Input: part model. Units: mm. Frame: model coordinates. A direction names the side the tool comes from. Coordinates: 2 decimals unless noted, no trailing zeros. Write each loop counter-clockwise with the first axis right and the second up, starting at its lowest first coordinate (ties: lowest second). Pieces come first, ordered by that corner, then holes.
from build123d import *

# Parameters (mm, degrees)
SKETCH_1_R          = 30.47
EXTRUDE_1_DEPTH     = 13
SKETCH_2_R          = 33.47
EXTRUDE_2_DEPTH     = 1.5
EXTRUDE_START       = 1.5
SKETCH_3_R          = 33.47
EXTRUDE_3_DEPTH     = 1.5
SKETCH_4_R          = 5
CUT_EXTRUDE_1_DEPTH = 50.964805614
SKETCH_5_R          = 11
CUT_EXTRUDE_2_DEPTH = 5


with BuildPart() as part:
    # 草图1 → 凸台-拉伸1 (new body)
    with BuildSketch(Plane.XY):
        with Locations(Location((0, 0, 0), (0, 0, 180))):
            Circle(SKETCH_1_R)
    extrude(amount=EXTRUDE_1_DEPTH)

    # 草图2 → 凸台-拉伸2 (add)
    with BuildSketch(Plane.XY.offset(13)):
        Circle(SKETCH_2_R)
    extrude(amount=EXTRUDE_2_DEPTH)

    # 草图3 → 凸台-拉伸3 (add)
    with BuildSketch(Plane(origin=(0, 0, 0), x_dir=(-1, 0, 0), z_dir=(0, 0, -1)).offset(EXTRUDE_START)):
        with Locations(Location((0, 0, 0), (0, 0, 180))):
            Circle(SKETCH_3_R)
    extrude(amount=-EXTRUDE_3_DEPTH)

    # 草图4 → 切除-拉伸1 (cut, through all)
    with BuildSketch(Plane.XY.offset(14.5)):
        Circle(SKETCH_4_R)
    extrude(amount=-CUT_EXTRUDE_1_DEPTH, mode=Mode.SUBTRACT)

    # 草图5 → 切除-拉伸2 (cut)
    with BuildSketch(Plane.XY.offset(14.5)):
        Circle(SKETCH_5_R)
    extrude(amount=-CUT_EXTRUDE_2_DEPTH, mode=Mode.SUBTRACT)


solid = part.part
Item 1: Section query C-C, the plane z = 11. Return loops of the section in (x, y).
Item 2: Pull-direction query (X, two-part tool) for faces 1 (the face through (-1.08, -4.88, 4.08)), 2 (the face through (-7.256, 32.674, -0.76)), 3 (the face through (-2.38, -10.74, 12.04)), 4 (the face through (-8, 8, 14.5)); classes: released by +X, released by -X, zero draft, split by the parting line, or undercut.
Item 3: Pin query (flat end, axial travel): pin 1 Ø17.5 at (x, y) = (0, 0) entering from +Z; pin 2 Ø1 at (x, z) = (-17, 4) entering from -Y; pin 3 Ø24 at (x, y) = (-5, 5) entering from +Z; pin 4 Ø8 at (y, z) = (-21, 3) entering from -X. Return the tip coordinate at first contact, or that it passes through.
Item 4: Access query for faces 5 (the face through (2, -5, 9.5)), 6 (the face through (6.605, 29.745, 6.409)), 7 (the face through (0, 7, -1.5)). Directions: +Z, -Z, +X, -X, +Y, -Y. A direction counts if a zero-diameter tool reaches every point of the face in a straight line with its end or side. Return the directions, or none.
Item 5: Material intervals for line 1 (Y direction, x = 0, z = 13.2); line 2 (Y direction, x = 0, z = 5); line 3 (X direction, y = 4.5, z = 7.5), sorted ascending.
Item 6: Section query D-D, the plane x = 12. Return loops of the section in (y, z), then the cut area to 3 significant figures.
Item 7: Section query A-A, the plane x = 0. Return loops of the section in (y, z), then the cut area to 3 significant figures.
The answers:
1. outline: circle Ø60.94 at (0, 0); hole circle Ø22 at (0, 0)
2. face 1: undercut
2. face 2: split by the parting line
2. face 3: undercut
2. face 4: zero draft
3. pin 1: stops at z = 9.5
3. pin 2: stops at y = -25.62
3. pin 3: stops at z = 14.5
3. pin 4: stops at x = -27.99
4. face 5: +Z
4. face 6: none
4. face 7: -Z, +X, -X, +Y, -Y
5. line 1: y = -33.47 to -11, 11 to 33.47
5. line 2: y = -30.47 to -5, 5 to 30.47
5. line 3: x = -30.14 to -2.18, 2.18 to 30.14
6. outline: (-31.24, -1.5) - (31.24, -1.5) - (31.24, 0) - (28.01, 0) - (28.01, 13) - (31.24, 13) - (31.24, 14.5) - (-31.24, 14.5) - (-31.24, 13) - (-28.01, 13) - (-28.01, 0) - (-31.24, 0) - close
6. area: 916 mm2
7. outline: (-33.47, -1.5) - (-5, -1.5) - (-5, 9.5) - (-11, 9.5) - (-11, 14.5) - (-33.47, 14.5) - (-33.47, 13) - (-30.47, 13) - (-30.47, 0) - (-33.47, 0) - close; (5, -1.5) - (33.47, -1.5) - (33.47, 0) - (30.47, 0) - (30.47, 13) - (33.47, 13) - (33.47, 14.5) - (11, 14.5) - (11, 9.5) - (5, 9.5) - close
7. area: 773 mm2
